Design review of the part built by this model. Coordinates are the model's own, in mm. Face numbers are marked on the shaded views. A direction names the side the tool comes from. Round coordinates to 2 decimals unless told otherwise and drop trailing zeros. Order: outer loops, then holes, each group sorted by start corner. A loop starts at its lowest first (then second) coordinate and runs counter-clockwise, first axis right, second up. Notation, with made-up numbers: (26, 47.5) - (48, 47.5) arc R17 cw to (48, 58.5) - close; hole circle Ø2 at (44, 53.5). An arc over 180 degrees is marked (long way). Use CSV: the item, a comma, the result in double quotes.
from build123d import *

# Parameters (mm, degrees)
BOSS_EXTRUDE1_DEPTH           = 7.62
BOSS_EXTRUDE2_START           = 2.54
SKETCH3_R                     = 1.27
BOSS_EXTRUDE2_DEPTH           = 2.54
TAP_DRILL_FOR_6_32_TAP1_D     = 2.7051
TAP_DRILL_FOR_6_32_TAP1_DEPTH = 7.62
TAP_DRILL_FOR_6_32_TAP1_TIP   = 0.81269403


with BuildPart() as part:
    # Sketch2 → Boss-Extrude1 (new body)
    with BuildSketch(Plane(origin=(0, 0, 0), x_dir=(1, 0, 0), z_dir=(0, 1, 0))):
        with BuildLine():
            Line((-7.447659431, 10.287), (7.447659431, 10.287))
            ThreePointArc((7.447659431, 10.287), (12.233908558, 3.409029391), (11.694348678, -4.953))
            Line((11.694348678, -4.953), (18.044348678, -4.953))
            Line((18.044348678, -4.953), (18.044348678, -7.747))
            Line((18.044348678, -7.747), (10.063497951, -7.747))
            Line((10.063497951, -7.747), (6.573400262, -7.747))
            ThreePointArc((6.573400262, -7.747), (10.16, 0), (6.573400262, 7.747))
            Line((6.573400262, 7.747), (-6.573400262, 7.747))
            ThreePointArc((-6.573400262, 7.747), (-10.16, 0), (-6.573400262, -7.747))
            Line((-6.573400262, -7.747), (-10.063497951, -7.747))
            Line((-10.063497951, -7.747), (-18.044348678, -7.747))
            Line((-18.044348678, -7.747), (-18.044348678, -4.953))
            Line((-18.044348678, -4.953), (-11.694348678, -4.953))
            ThreePointArc((-11.694348678, -4.953), (-12.233908558, 3.409029391), (-7.447659431, 10.287))
        make_face()
    extrude(amount=BOSS_EXTRUDE1_DEPTH)

    # Sketch3 → Boss-Extrude2 (add)
    with BuildSketch(Plane.XZ.offset(BOSS_EXTRUDE2_START)):
        with BuildLine():
            Line((7.447659431, -10.287), (-7.447659431, -10.287))
            ThreePointArc((-7.447659431, -10.287), (-12.568470361, -1.823061379), (-10.063497951, 7.747))
            Line((-10.063497951, 7.747), (10.063497951, 7.747))
            ThreePointArc((10.063497951, 7.747), (12.568470361, -1.823061379), (7.447659431, -10.287))
        make_face()
        with Locations(Location((0, 0, 0), (0, 0, 270))):
            Circle(SKETCH3_R, mode=Mode.SUBTRACT)
    extrude(amount=-BOSS_EXTRUDE2_DEPTH)

    # Tap Drill for #6-32 Tap1
    with Locations(Plane(origin=(0, 0, 4.953), x_dir=(-1, 0, 0), z_dir=(0, 0, -1))):
        with Locations((-14.488348678, 3.81), (14.488348678, 3.81)):
            Hole(TAP_DRILL_FOR_6_32_TAP1_D / 2, depth=TAP_DRILL_FOR_6_32_TAP1_DEPTH)
            with Locations((0, 0, -(TAP_DRILL_FOR_6_32_TAP1_DEPTH + TAP_DRILL_FOR_6_32_TAP1_TIP / 2))):  # 118° drill point
                Cone(0, TAP_DRILL_FOR_6_32_TAP1_D / 2, TAP_DRILL_FOR_6_32_TAP1_TIP, mode=Mode.SUBTRACT)


solid = part.part
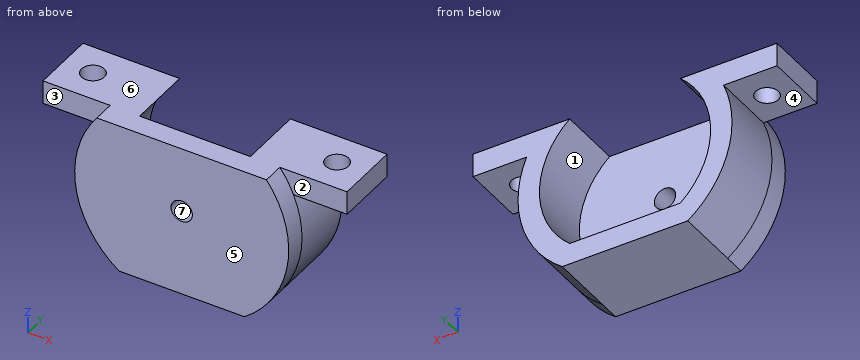
1) Insertion check: pin 1 Ø3 at (x, z) = (13.5, 6) entering from -Y; pin 2 Ø5 at (x, y) = (-13.5, 2.5) entering from -Z; pin 3 Ø1.5 at (y, z) = (-1, 4.5) entering from +X; pin 4 Ø2 at (x, y) = (14.49, 3.81) entering from +Z (3 decimals). Each pin has a flat end and moves straight along its axis. Give the tip position at first contact, or say it passes through.
Data:
pin 1,"stops at y = 0"
pin 2,"stops at z = -6.35"
pin 3,"stops at x = 12.13"
pin 4,"passes through"
2) We need section D-D (y = -0.5). Give the boundary of the cut face in (x, z), then the cut area to 3 significant figures.
Data:
outline,"(-10.06, 7.75) arc R12.7 ccw to (-7.45, -10.29) - (7.45, -10.29) arc R12.7 ccw to (10.06, 7.75) - close; hole circle Ø2.54 at (0, 0)"
area,"408 mm2"
3) We need section B-B (z = 0). Give the boundary of the cut face in (x, y).
Data:
outline,"(-12.7, -2.54) - (-1.27, -2.54) - (-1.27, 0) - (-10.16, 0) - (-10.16, 7.62) - (-12.7, 7.62) - close; (1.27, -2.54) - (12.7, -2.54) - (12.7, 7.62) - (10.16, 7.62) - (10.16, 0) - (1.27, 0) - close"
4) To check wall thickness, follow L1, parallel to X at y = -1.95, z = 0; L2, parallel to Z at x = -0.5, y = 6; L3, parallel to X at y = 5, z = 7.25. State the ranges of each line that lie inside material, in increasing order. Write a range as from..to.
Data:
L1,"x = -12.7..-1.27, 1.27..12.7"
L2,"z = -10.29..-7.75"
L3,"x = -18.04..-15.13, -13.85..-7.12, 7.12..13.85, 15.13..18.04"
5) We need section C-C (y = 3.81). Give the boundary of the cut face in (x, z).
Data:
outline,"(-18.04, 4.95) - (-15.84, 4.95) - (-15.84, 7.75) - (-18.04, 7.75) - close; (-13.14, 4.95) - (-11.69, 4.95) arc R12.7 ccw to (-7.45, -10.29) - (7.45, -10.29) arc R12.7 ccw to (11.69, 4.95) - (13.14, 4.95) - (13.14, 7.75) - (6.57, 7.75) arc R10.16 cw to (6.57, -7.75) - (-6.57, -7.75) arc R10.16 cw to (-6.57, 7.75) - (-13.14, 7.75) - close; (15.84, 4.95) - (18.04, 4.95) - (18.04, 7.75) - (15.84, 7.75) - close"
6) We need section A-A (x = 0). Give the boundary of the cut face in (y, z).
Data:
outline,"(-2.54, -10.29) - (7.62, -10.29) - (7.62, -7.75) - (0, -7.75) - (0, -1.27) - (-2.54, -1.27) - close; (-2.54, 1.27) - (0, 1.27) - (0, 7.75) - (-2.54, 7.75) - close"
7) The part is to be moulded in two halves that separate along Z. For the marked faces 5, 6 and 7, say which applies: +Z half, -Z half, draft (parallel to the pull), parting line (faces both ways), or undercut.
Data:
face 5,"draft"
face 6,"+Z half"
face 7,"undercut"
8) For the marked faces 1, 2, 3 and 4, list the 3-axis set-ups (+Z, -Z, +X, -X, +Y, -Y) from which the entire face can be reached by the end or side of a thin tool; tool diameter is ignored.
Data:
face 1,"+Y"
face 2,"+Z, +X, -Y"
face 3,"+Z, -X, -Y"
face 4,"-X, +Y, -Y"
